```python
from build123d import *

# Parameters (mm, degrees)
F1_DEPTH = 25


with BuildPart() as f1:
    # F0 (on Front) → F1 (new body)
    with BuildSketch(Plane.XZ):
        Polygon((60.819678, 52.930329), (0, 0), (-60.819678, 52.930329), (-32.418031, 0), (-70.57377, -70.430331), (-32.418031, -23.094265), (32.418031, -23.094265), (70.57377, -70.430331), (32.418031, 0), align=None)
    extrude(amount=F1_DEPTH)

    # F1_face (on face) → F4 section 0
    with BuildSketch(Plane(origin=(0, -25, -3.53806), x_dir=(1, 0, 0), z_dir=(0, -1, 0)), mode=Mode.PRIVATE) as f4_s0:
        Polygon((-60.819678, 56.468389), (-32.418031, 3.53806), (-70.57377, -66.892271), (-32.418031, -19.556205), (32.418031, -19.556205), (70.57377, -66.892271), (32.418031, 3.53806), (60.819678, 56.468389), (0, 3.53806), align=None)
    loft([f4_s0.sketch, Vertex(0, -100, 0)])


solid = f1.part
```
Verification items for the finished model (mm, model axes). A direction names the side the tool comes from. Give positions to 0.01 mm unless a question says otherwise; leave off trailing zeros. Order: outer loops, then holes, each group sorted by start corner. A loop starts at its lowest first (then second) coordinate and runs counter-clockwise, first axis right, second up. Notation, with made-up numbers: (32, 87.25) - (40, 87.25) arc R30 cw to (40, 125.25) - close; hole circle Ø4 at (41, 87.25). An arc over 180 degrees is marked (long way). Answer as CSV lines item,"result". Start each with the question number.
Item 1: Material ranges on L1, parallel to X at y = -49.5, z = 20.5; L2, parallel to X at y = -74.5, z = 9; L3, parallel to Z at x = 35, y = -32.5, recorded low to high.
Item 2: Section check B-B, the plane z = 45. Record the boundary of the cut face in (x, y).
Item 3: Access from +Z, -Z, +X, -X, +Y, -Y to the whole of each face (thin tool, end or side, straight path). Record for faces 1 (the face through (-23.226, -39.589, 20.214)), 2 (the face through (35.9, -46.4, -23.5)), 3 (the face through (0, -12, -23.094)), 4 (the face through (-0.45, -54.69, -13.95)).
Item 4: Mould release check, pull along Y, two halves, no side actions. Record for faces 5 (the face through (34.368, -48.786, -30.944)), 6 (the face through (-51.229, -12.325, -34.722)), 7 (the face through (30.968, -48.786, 16.459)), 8 (the face through (-34.348, -51.564, -31.554)): released by +Y, released by -Y, zero draft, split by the parting line, or undercut.
Item 5: Gauge pin test, flat ends, axial feed: pin 1 (3 mm diameter, centred on x = -20, y = -47, fed in from -Z); pin 2 (10 mm diameter, centred on x = 29.5, y = -42, fed in from -Z); pin 3 (7.5 mm diameter, centred on x = 15.5, y = -7.5, fed in from -Z). Record the tip position at first contact, or that the pin passes through.
Item 6: Section check A-A, the plane x = -38. Record the boundary of the cut face in (y, z), plus the area to 3 significant figures.
Item 7: Section check C-C, the plane y = -10. Record the boundary of the cut face in (x, z), plus the area to 3 significant figures.
Item 8: Section check D-D, the plane x = -55.5. Record the boundary of the cut face in (y, z), plus the area to 3 significant figures.
Filled in:
1,L1,"-32.83 to -23.56, 23.56 to 32.83"
1,L2,"-15.85 to -10.34, 10.34 to 15.85"
1,L3,"-28.01 to -10.75, 10.85 to 30.46"
2,outline,"(-56.56, -25) - (-51.71, -36.24) - (-51.71, 0) - (-56.56, 0) - close; (51.71, -36.24) - (56.56, -25) - (56.56, 0) - (51.71, 0) - close"
3,face 1,"+Z, +Y, -Y"
3,face 2,"+X, -Y"
3,face 3,"-Z, +Y"
3,face 4,"-Z"
4,face 5,"undercut"
4,face 6,"zero draft"
4,face 7,"released by -Y"
4,face 8,"undercut"
5,pin 1,"z = -16.78"
5,pin 2,"z = -29.66"
5,pin 3,"z = -23.09"
6,outline,"(-59.62, -37.92) - (-25, -30.02) - (0, -30.02) - (0, -10.3) - (-25, -10.3) - close; (-53.14, 33.07) - (-25, 10.4) - (0, 10.4) - (0, 33.07) - close"
6,area,"1,720 mm^2"
7,outline,"(-70.57, -70.43) - (-32.42, -23.09) - (32.42, -23.09) - (70.57, -70.43) - (32.42, 0) - (60.82, 52.93) - (0, 0) - (-60.82, 52.93) - (-32.42, 0) - close"
7,area,"4,090 mm^2"
8,outline,"(-41.02, -55.39) - (-25, -51.73) - (0, -51.73) - (0, -42.61) - (-25, -42.61) - close; (-31.56, 48.3) - (-25, 43.02) - (0, 43.02) - (0, 48.3) - close"
8,area,"451 mm^2"
